Check sheet for the modelled part. Datum: model origin and axes. Units: mm. Round coordinates to 2 decimals unless told otherwise and drop trailing zeros. Write each loop counter-clockwise with the first axis right and the second up, starting at its lowest first coordinate (ties: lowest second). Pieces come first, ordered by that corner, then holes. Notation, with made-up numbers: M 31,-13.5 L 61,-13.5 A22 cw 61,15.5 Z; hole C 28,6 d10. An arc over 180 degrees is marked long. One line per item, written item: value.
Autodesk Inventor part; units mm, degrees
ref_plane "YZ Plane" through (0, 0, 0) normal (1, 0, 0) x (0, 1, 0)
ref_plane "XZ Plane" through (0, 0, 0) normal (0, 1, 0) x (-1, 0, 0)
ref_plane "XY Plane" through (0, 0, 0) normal (0, 0, 1) x (1, 0, 0)
sketch "Sketch1" plane through (0, 0, 0) normal (0, 1, 0) x (-1, 0, 0)
  circle A0 centre (0, 0) radius 25.4
  dimension "d0" = 50.8
extrude "Extrusion1" add sketch "Sketch1" along normal blind 12.7
sketch "Sketch2" plane through (0, 12.7, 0) normal (0, 1, 0) x (1, 0, 0)
  circle A0 centre (0, 0) radius 19.05
  dimension "d3" = 38.1
extrude "Extrusion2" add sketch "Sketch2" along normal blind 12.7
fillet "Fillet1" radius 6.35 1 edges at (-19.05, 12.7, 0)
sketch "Sketch3" plane through (0, 25.4, 0) normal (0, 1, 0) x (1, 0, 0)
  circle A0 centre (0, 0) radius 25.4
  dimension "d7" = 50.8
extrude "Extrusion3" add sketch "Sketch3" along normal blind 12.7
fillet "Fillet2" radius 6.35 1 edges at (-19.05, 25.4, 0)
Q1. Sectioned sample at C-C on y = 8.5. Enter the section's corners in (x, z), and give its area (3 significant figures).
Completed:
outline: C 0,0 d50.8
area: 2,030 mm^2
Q2. Sectioned sample at D-D on y = 17.5. Enter the section's corners in (x, z).
Completed:
outline: C 0,0 d38.48
Q3. Depth check by flat-ended pin: P1, Ø3, axis at y = 13.5, z = -0.5, coming from the +X side; P2, Ø12, axis at x = -18.5, y = 32.5, coming from the +Z side; P3, Ø2, axis at y = 33.5, z = 10, coming from the -X side; P4, Ø6, axis at x = -6.5, y = 26.5, coming from the +Z side. Enter the tip coordinate at first touch or a pass-through.
Completed:
P1: x = 25.4
P2: z = 22.11
P3: x = -23.75
P4: z = 25.16
Q4. Scan lines: line 1 (Y direction, x = -10, z = 23); line 2 (Y direction, x = -16.5, z = 11.5); line 3 (Z direction, x = -11, y = 8). Record each from-to range of solid material in increasing order. Write a range as [from, to].
Completed:
line 1: [0, 12.71], [25.39, 38.1]
line 2: [0, 15.53], [22.57, 38.1]
line 3: [-22.89, 22.89]
